Input: part model. Units: mm. Frame: model coordinates. Face numbers are marked on the shaded views. Round coordinates to 2 decimals unless told otherwise and drop trailing zeros. Loops run counter-clockwise (first coordinate to the right, second up) from the corner with the lowest first, then second, coordinate; pieces in that order, holes last. Notation, with made-up numbers: (-22, 19) - (17, 19) arc R30 ccw to (17, 55) - close; hole circle Ø2 at (48.5, 27). An arc over 180 degrees is marked (long way). One line per question, with ' | ' between items. Start each with the question number.
Item 1: First-contact query: pin 1 (10.5 mm diameter, centred on x = 36.5, y = 80, fed in from +Z); pin 2 (2.5 mm diameter, centred on y = 80, z = 11.25, fed in from +X). Flat tips, straight axial feed; report the tip coordinate or a pass-through.
Item 2: Section A-A, the plane x = 21. Return loops of the section in (y, z).
Item 3: Draft query along Y for the marked faces 1, 2, 3 and 4. Return one class per face: pulls with the +Y half, pulls with the -Y half, needs draft (parallel to the pull), parting line crosses it, or undercut.
Item 4: Material intervals for line 1 along Y through (x, z) = (21, 4.5); line 2 along X through (y, z) = (9, 3.75); line 3 along Y through (x, z) = (30, 8.5), sorted ascending.
Item 5: Section D-D, the plane z = 11.25. Give the number of separate pieces and of enclosed holes in the cut face, plus the area to 3 significant figures.
Item 6: Section B-B, the plane x = 10. Return loops of the section in (y, z), plus the area to 3 significant figures.
Item 7: Section C-C, the plane y = 110. Return loops of the section in (x, z), plus the area to 3 significant figures.
```python
from build123d import *

# Parameters (mm, degrees)
SKETCH1_W               = 60
SKETCH1_H               = 120
SKETCH1_R               = 2.5
BOSS_EXTRUDE1_DEPTH     = 15
FILLET1_R               = 3
SKETCH2_R               = 4.5
SKETCH2_R_2             = 1.5
CUT_EXTRUDE1_DEPTH      = 136
SKETCH2_3_R             = 11
SKETCH2_3_R_2           = 4.5
CUT_EXTRUDE2_DEPTH      = 7.5
CUT_EXTRUDE3_REACH      = 137
CUT_EXTRUDE3_END_RADIUS = 11
SKETCH3_R               = 1.5


with BuildPart() as part:
    # Sketch1 → Boss-Extrude1 (new body)
    with BuildSketch(Plane.XY):
        with Locations((30, 60)):
            Rectangle(SKETCH1_W, SKETCH1_H)
        with Locations((10, 110)):
            Circle(SKETCH1_R, mode=Mode.SUBTRACT)
        with Locations((30, 110)):
            Circle(SKETCH1_R, mode=Mode.SUBTRACT)
        with Locations((10, 90)):
            Circle(SKETCH1_R, mode=Mode.SUBTRACT)
        with Locations((10, 70)):
            Circle(SKETCH1_R, mode=Mode.SUBTRACT)
        with Locations((10, 10)):
            Circle(SKETCH1_R, mode=Mode.SUBTRACT)
        with Locations((30, 10)):
            Circle(SKETCH1_R, mode=Mode.SUBTRACT)
        with Locations((30, 50)):
            Circle(SKETCH1_R, mode=Mode.SUBTRACT)
        with Locations((10, 50)):
            Circle(SKETCH1_R, mode=Mode.SUBTRACT)
        with Locations((10, 30)):
            Circle(SKETCH1_R, mode=Mode.SUBTRACT)
        with Locations((30, 30)):
            Circle(SKETCH1_R, mode=Mode.SUBTRACT)
    extrude(amount=BOSS_EXTRUDE1_DEPTH)

    # Fillet1
    fillet1_edges = [part.edges().sort_by_distance(p)[0] for p in [
        (0, 120, 7.5),
        (60, 120, 7.5),
        (60, 0, 7.5),
        (0, 0, 7.5),
    ]]
    fillet(fillet1_edges, radius=FILLET1_R)

    # Sketch2 → Cut-Extrude1 (cut, through all)
    with BuildSketch(Plane.XY.offset(15)):
        with Locations((36.5, 80)):
            Circle(SKETCH2_R)
        with Locations((52, 95.5)):
            Circle(SKETCH2_R_2)
        with Locations((21, 95.5)):
            Circle(SKETCH2_R_2)
        with Locations((52, 64.5)):
            Circle(SKETCH2_R_2)
        with Locations((21, 64.5)):
            Circle(SKETCH2_R_2)
    extrude(amount=-CUT_EXTRUDE1_DEPTH, mode=Mode.SUBTRACT)

    # Sketch2<3> → Cut-Extrude2 (cut)
    with BuildSketch(Plane.XY.offset(15)):
        with Locations((36.5, 80)):
            Circle(SKETCH2_3_R)
        with Locations((36.5, 80)):
            Circle(SKETCH2_3_R_2, mode=Mode.SUBTRACT)
    extrude(amount=-CUT_EXTRUDE2_DEPTH, mode=Mode.SUBTRACT)

    # Cut-Extrude3: up to this cylinder (the profile starts outside it)
    cut_extrude3_end = Plane(origin=(36.5, 80, 11.25), z_dir=(0, 0, 1)) * Cylinder(CUT_EXTRUDE3_END_RADIUS, 297, mode=Mode.PRIVATE)
    # Sketch3 → Cut-Extrude3 (cut, up to the surface)
    with BuildSketch(Plane(origin=(60, 0, 0), x_dir=(0, 0, -1), z_dir=(1, 0, 0)), mode=Mode.PRIVATE) as cut_extrude3_sk1:
        with Locations((-11.25, 80)):
            Circle(SKETCH3_R)
    cut_extrude3_tool1 = extrude(cut_extrude3_sk1.sketch, amount=-CUT_EXTRUDE3_REACH, mode=Mode.PRIVATE) - cut_extrude3_end
    add(cut_extrude3_tool1.solids().sort_by_distance((60, 80, 11.25))[0], mode=Mode.SUBTRACT)


solid = part.part
```
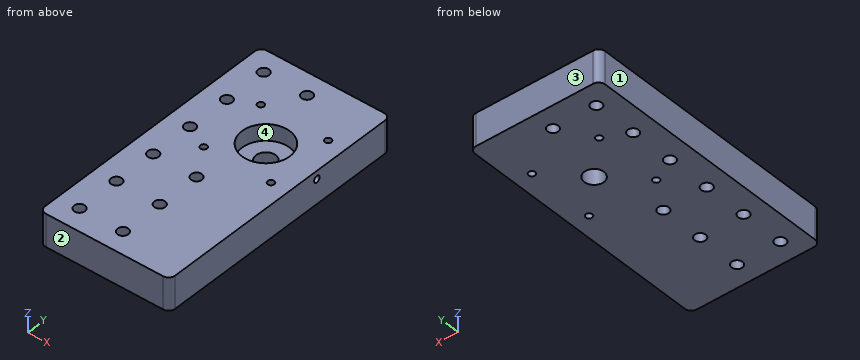
Return value:
1) pin 1: z = 7.5 | pin 2: x = 25.57
2) outline: (0, 0) - (63, 0) - (63, 15) - (0, 15) - close; (66, 0) - (94, 0) - (94, 15) - (66, 15) - close; (97, 0) - (120, 0) - (120, 15) - (97, 15) - close
3) face 1: needs draft | face 2: pulls with the -Y half | face 3: pulls with the +Y half | face 4: undercut
4) line 1: 0 to 63, 66 to 94, 97 to 120 | line 2: 0 to 7.71, 12.29 to 27.71, 32.29 to 60 | line 3: 0 to 7.5, 12.5 to 27.5, 32.5 to 47.5, 52.5 to 71.13, 88.87 to 107.5, 112.5 to 120
5) separate pieces: 1 | enclosed holes: 14 | area: 6,550 mm2
6) outline: (0, 0) - (7.5, 0) - (7.5, 15) - (0, 15) - close; (12.5, 0) - (27.5, 0) - (27.5, 15) - (12.5, 15) - close; (32.5, 0) - (47.5, 0) - (47.5, 15) - (32.5, 15) - close; (52.5, 0) - (67.5, 0) - (67.5, 15) - (52.5, 15) - close; (72.5, 0) - (87.5, 0) - (87.5, 15) - (72.5, 15) - close; (92.5, 0) - (107.5, 0) - (107.5, 15) - (92.5, 15) - close; (112.5, 0) - (120, 0) - (120, 15) - (112.5, 15) - close | area: 1,350 mm2
7) outline: (0, 0) - (7.5, 0) - (7.5, 15) - (0, 15) - close; (12.5, 0) - (27.5, 0) - (27.5, 15) - (12.5, 15) - close; (32.5, 0) - (60, 0) - (60, 15) - (32.5, 15) - close | area: 750 mm2
